Input: part model. Units: mm. Frame: model coordinates. A direction names the side the tool comes from. Give positions to 0.01 mm unless a question says otherwise; leave off trailing zeros. Loops run counter-clockwise (first coordinate to the right, second up) from the corner with the lowest first, then second, coordinate; pieces in that order, holes last. Notation, with made-up numbers: M 8,30 L 12,30 A18 ccw 12,38 Z; hole C 54.25,34 d3. An arc over 180 degrees is marked long. One line per item, written item: value. Start each with the question number.
(1) Section B-B on x = -22. Output: boundary loops of the cut face in (y, z).
(2) Pull-direction query (Y, two-part tool) for faces 1 (the flat face through (23, 11, 1)), 2 (the flat face through (30, -26, 2)), 3 (the flat face through (25.5, -21, 1)); classes: released by +Y, released by -Y, zero draft, split by the parting line, or undercut.
(3) Pin query (flat end, axial travel): P1, Ø0.5, axis at x = 24, z = 0.5, coming from the -Y side; P2, Ø5, axis at x = -26, y = -1.5, coming from the +Z side; P3, Ø14, axis at x = 14.5, y = -5.5, coming from the +Z side. Return the tip coordinate at first contact, or that it passes through.
(4) Section C-C on y = -3.5. Output: boundary loops of the cut face in (x, z).
(5) Section A-A on y = 10. Output: boundary loops of the cut face in (x, z), plus the area to 3 significant figures.
(6) Ray query, line 1 along X through (y, z) = (-1, 1.9); line 2 along X through (y, z) = (7, 2.85); line 3 along Y through (x, z) = (9.5, 0.55). Return the intervals inside material, ascending. Write a range as from..to.
(7) Section D-D on x = 14.5. Output: boundary loops of the cut face in (y, z).
(8) Access query for faces 4 (the flat face through (24, -3, 1)), 5 (the flat face through (19, -12, 1)), 6 (the flat face through (20, 25, 4)), 7 (the flat face through (-30, -26, 2)), 8 (the flat face through (19, 19, 1)). Directions: +Z, -Z, +X, -X, +Y, -Y. A direction counts if a zero-diameter tool reaches every point of the face in a straight line with its end or side. Return the directions, or none.
```python
from build123d import *

# Parameters (mm, degrees)
SKICA1_W                    = 67
SKICA1_H                    = 50
P_IDAT_VYSUNUT_M1_DEPTH     = 3
ODEBRAT_VYSUNUT_M1_DEPTH    = 1
SKICA3_W                    = 8
SKICA3_H                    = 8
ODEBRAT_VYSUNUT_M2_DEPTH    = 4
VYSUNOUT_TENKOST_NN_1_DEPTH = 1
VYSUNOUT_TENKOST_NN_2_DEPTH = 5
SKICA6_W                    = 12
SKICA6_H                    = 4
ODEBRAT_VYSUNUT_M3_DEPTH    = 4
SKICA7_W                    = 5
SKICA7_H                    = 5
ODEBRAT_VYSUNUT_M5_DEPTH    = 1
P_IDAT_START                = -1
SKICA8_W                    = 1.6
SKICA8_H                    = 0.8
SKICA8_H_2                  = 2.4
P_IDAT_VYSUNUT_M3_DEPTH     = 1


with BuildPart() as part:
    # Skica1 → Přidat vysunutím1 (new body)
    with BuildSketch(Plane.XY):
        Rectangle(SKICA1_W, SKICA1_H)
    extrude(amount=P_IDAT_VYSUNUT_M1_DEPTH)

    # Skica2 → Odebrat vysunutím1 (cut)
    with BuildSketch(Plane.XY.offset(3)):
        Polygon((-25.5, -22), (-30.5, -17), (-30.5, 17), (-25.5, 22), (25.5, 22), (30.5, 17), (30.5, -17), (25.5, -22), align=None)
    extrude(amount=-ODEBRAT_VYSUNUT_M1_DEPTH, mode=Mode.SUBTRACT)

    # Skica3 → Odebrat vysunutím2 (cut, through all)
    with BuildSketch(Plane(origin=(0, 0, 0), x_dir=(-1, 0, 0), z_dir=(0, 0, -1))):
        with Locations((20, -3)):
            Rectangle(SKICA3_W, SKICA3_H)
        with Locations((-20, -3)):
            Rectangle(SKICA3_W, SKICA3_H)
        Polygon((25.5, -25), (-25.5, -25), (-25.5, -12), (-12, -12), (-12, 15), (12, 15), (12, -12), (25.5, -12), align=None)
    extrude(amount=-ODEBRAT_VYSUNUT_M2_DEPTH, mode=Mode.SUBTRACT)

    # Skica4 → Vysunout tenkostěnný1 (add)
    with BuildSketch(Plane.XY.offset(2)):
        Polygon((-12, -12), (-12, 15), (12, 15), (12, -12), (13, -12), (13, 16), (-13, 16), (-13, -12), align=None)
    extrude(amount=VYSUNOUT_TENKOST_NN_1_DEPTH)

    # Skica5 → Vysunout tenkostěnný2 (add)
    with BuildSketch(Plane(origin=(0, 0, 0), x_dir=(-1, 0, 0), z_dir=(0, 0, -1))):
        Polygon((-25.5, -25), (-33.5, -25), (-33.5, 25), (33.5, 25), (33.5, -25), (25.5, -25), (25.5, -26), (34.5, -26), (34.5, 26), (-34.5, 26), (-34.5, -26), (-25.5, -26), align=None)
    extrude(amount=-VYSUNOUT_TENKOST_NN_2_DEPTH)

    # Skica6 → Odebrat vysunutím3 (cut, through all)
    with BuildSketch(Plane.XY.offset(2)):
        with Locations((0, 24)):
            Rectangle(SKICA6_W, SKICA6_H)
    extrude(amount=ODEBRAT_VYSUNUT_M3_DEPTH, mode=Mode.SUBTRACT)

    # Skica7 → Odebrat vysunutím5 (cut)
    with BuildSketch(Plane(origin=(0, 0, 0), x_dir=(-1, 0, 0), z_dir=(0, 0, -1))):
        with Locations((-28, 18.5)):
            Rectangle(SKICA7_W, SKICA7_H)
        with Locations((-18.5, 18.5)):
            Rectangle(SKICA7_W, SKICA7_H)
        Polygon((-25.5, 15.99), (-25.5, 13.5), (-28, 13.5), (-28, 6), (-25.5, 6), (-25.5, 8.49), (-21, 8.49), (-21, 6), (-18.5, 6), (-18.5, 13.5), (-21, 13.5), (-21, 15.99), align=None)
        Polygon((21, 13.5), (18.5, 13.5), (18.5, 6), (21, 6), (21, 8.49), (25.5, 8.49), (25.5, 6), (28, 6), (28, 13.5), (25.5, 13.5), (25.5, 15.99), (21, 15.99), align=None)
        with Locations((18.5, 18.5)):
            Rectangle(SKICA7_W, SKICA7_H)
        with Locations((28, 18.5)):
            Rectangle(SKICA7_W, SKICA7_H)
        Polygon((-11.2, 23.3), (-11.2, 17.7), (-7.2, 17.7), (-7.2, 18.5), (-6.4, 18.5), (-6.4, 20.1), (-7.2, 20.1), (-7.2, 20.9), (-6.4, 20.9), (-6.4, 22.5), (-7.2, 22.5), (-7.2, 23.3), align=None)
        Polygon((-1.6, 23.3), (-4.8, 23.3), (-4.8, 22.5), (-5.6, 22.5), (-5.6, 18.5), (-4.8, 18.5), (-4.8, 17.7), (-1.6, 17.7), (-1.6, 18.5), (-0.8, 18.5), (-0.8, 22.5), (-1.6, 22.5), align=None)
        Polygon((0.8, 23.3), (0.8, 22.5), (0, 22.5), (0, 18.5), (0.8, 18.5), (0.8, 17.7), (4, 17.7), (4, 18.5), (4.8, 18.5), (4.8, 22.5), (4, 22.5), (4, 23.3), align=None)
        Polygon((5.6, 17.7), (5.6, 23.3), (7.2, 23.3), (7.2, 22.5), (8, 22.5), (8, 21.7), (8.8, 21.7), (8.8, 22.5), (9.6, 22.5), (9.6, 23.3), (11.2, 23.3), (11.2, 17.7), (9.6, 17.7), (9.6, 19.3), (8.8, 19.3), (8.8, 18.5), (8, 18.5), (8, 19.3), (7.2, 19.3), (7.2, 17.7), align=None)
    extrude(amount=-ODEBRAT_VYSUNUT_M5_DEPTH, mode=Mode.SUBTRACT)

    # Skica8 → Přidat vysunutím3 (add)
    with BuildSketch(Plane(origin=(0, 0, 0), x_dir=(-1, 0, 0), z_dir=(0, 0, -1)).offset(P_IDAT_START)):
        with Locations((-8.8, 21.3)):
            Rectangle(SKICA8_W, SKICA8_H)
        with Locations((-8.8, 19.7)):
            Rectangle(SKICA8_W, SKICA8_H)
        with Locations((-3.2, 20.5)):
            Rectangle(SKICA8_W, SKICA8_H_2)
        with Locations((2.4, 20.5)):
            Rectangle(SKICA8_W, SKICA8_H_2)
    extrude(amount=P_IDAT_VYSUNUT_M3_DEPTH)


solid = part.part
```
Output values:
1. outline: M -12,0 L -7,0 L -7,2 L -12,2 Z; M 1,0 L 8.49,0 L 8.49,1 L 15.99,1 L 15.99,0 L 26,0 L 26,5 L 25,5 L 25,3 L 22,3 L 22,2 L 1,2 Z
2. face 1: undercut
2. face 2: released by -Y
2. face 3: zero draft
3. P1: stops at y = -12
3. P2: stops at z = 2
3. P3: stops at z = 3
4. outline: M -34.5,0 L -24,0 L -24,2 L -30.5,2 L -30.5,3 L -33.5,3 L -33.5,5 L -34.5,5 Z; M -16,0 L -12,0 L -12,3 L -13,3 L -13,2 L -16,2 Z; M 12,0 L 16,0 L 16,2 L 13,2 L 13,3 L 12,3 Z; M 24,0 L 34.5,0 L 34.5,5 L 33.5,5 L 33.5,3 L 30.5,3 L 30.5,2 L 24,2 Z
5. outline: M -34.5,0 L -28,0 L -28,1 L -18.5,1 L -18.5,0 L -12,0 L -12,3 L -13,3 L -13,2 L -30.5,2 L -30.5,3 L -33.5,3 L -33.5,5 L -34.5,5 Z; M 12,0 L 18.5,0 L 18.5,1 L 28,1 L 28,0 L 34.5,0 L 34.5,5 L 33.5,5 L 33.5,3 L 30.5,3 L 30.5,2 L 13,2 L 13,3 L 12,3 Z
5. area: 85.0 mm²
6. line 1: x = -34.5..-24, -16..-12, 12..16, 24..34.5
6. line 2: x = -34.5..-30.5, -13..-12, 12..13, 30.5..34.5
6. line 3: y = 15..17.7, 19.3..20.1, 20.9..21.7, 23.3..26
7. outline: M -12,0 L 26,0 L 26,5 L 25,5 L 25,3 L 22,3 L 22,2 L -12,2 Z
8. face 4: +Z, -Z
8. face 5: +Z, -Z, -Y
8. face 6: +Z
8. face 7: +Z, -Z, +X, -X, -Y
8. face 8: -Z
